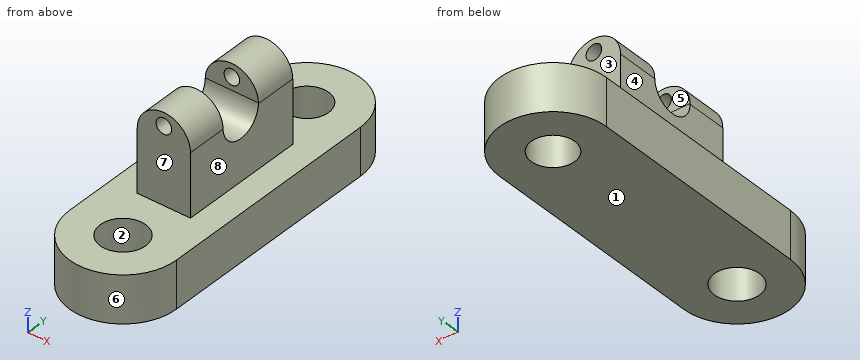
from build123d import *

# Parameters (mm, degrees)
F0_R      = 9.207917
F0_R_2    = 8.8097795002
F1_DEPTH  = 19.05
F2_W      = 21.5854309499
F2_H      = 51.5172295272
F3_DEPTH  = 25.4
F5_DEPTH  = 53.34
F7_DEPTH  = 25.4
F8_DEPTH  = 25.4
F9_W      = 17.8439589217
F9_H      = 25.0391028821
F10_DEPTH = 25.4
F11_DEPTH = 25.4
F12_R     = 3.1560406616
F13_DEPTH = 76.2


with BuildPart() as f1:
    # F0 (on Top) → F1 (new body)
    with BuildSketch(Plane.XY):
        with BuildLine():
            ThreePointArc((21.6257235091, 46.3394257879), (0, 67.965149297), (-21.6257235091, 46.3394257879))
            Line((-21.6257235091, 46.3394257879), (-21.6257235091, -46.3394257879))
            ThreePointArc((-21.6257235091, -46.3394257879), (0, -67.965149297), (21.6257235091, -46.3394257879))
            Line((21.6257235091, -46.3394257879), (21.6257235091, 46.3394257879))
        make_face()
        with Locations((0, -46.3394257879)):
            Circle(F0_R, mode=Mode.SUBTRACT)
        with Locations((0, 46.3394257879)):
            Circle(F0_R_2, mode=Mode.SUBTRACT)
    extrude(amount=F1_DEPTH)

    # F2 (on face) → F3 (join)
    with BuildSketch(Plane.XY.offset(19.05)):
        Rectangle(F2_W, F2_H)
    extrude(amount=F3_DEPTH)

    # F4 (on face) → F5 (join)
    with BuildSketch(Plane.XZ.offset(25.7586147636)):
        with BuildLine():
            Line((0, 44.45), (10.792715475, 44.45))
            ThreePointArc((10.792715475, 44.45), (0, 55.242715475), (-10.792715475, 44.45))
            Line((-10.792715475, 44.45), (0, 44.45))
        make_face()
    extrude(amount=-F5_DEPTH)

    # F6 (on Right) → F7 (cut)
    with BuildSketch(Plane.YZ):
        Polygon((25.7586147636, 59.1440834105), (25.7586147636, 44.753793627), (25.7586147636, 35.5440117419), (39.5732931793, 35.5440117419), (39.5732931793, 59.1440834105), align=None)
    extrude(amount=-F7_DEPTH, mode=Mode.SUBTRACT)

    # F6 (on Right) → F8 (cut)
    with BuildSketch(Plane.YZ):
        Polygon((25.7586147636, 59.1440834105), (25.7586147636, 44.753793627), (25.7586147636, 35.5440117419), (39.5732931793, 35.5440117419), (39.5732931793, 59.1440834105), align=None)
    extrude(amount=F8_DEPTH, mode=Mode.SUBTRACT)

    # F9 (on Right) → F10 (cut)
    with BuildSketch(Plane.YZ):
        with Locations((-0.4317085259, 57.2733450681)):
            Rectangle(F9_W, F9_H)
        with BuildLine():
            Line((8.490270935, 44.753793627), (-9.3536879867, 44.753793627))
            ThreePointArc((-9.3536879867, 44.753793627), (-0.4317085259, 35.8318141662), (8.490270935, 44.753793627))
        make_face()
    extrude(amount=-F10_DEPTH, mode=Mode.SUBTRACT)

    # F9 (on Right) → F11 (cut)
    with BuildSketch(Plane.YZ):
        with Locations((-0.4317085259, 57.2733450681)):
            Rectangle(F9_W, F9_H)
        with BuildLine():
            Line((8.490270935, 44.753793627), (-9.3536879867, 44.753793627))
            ThreePointArc((-9.3536879867, 44.753793627), (-0.4317085259, 35.8318141662), (8.490270935, 44.753793627))
        make_face()
    extrude(amount=F11_DEPTH, mode=Mode.SUBTRACT)

    # F12 (on face) → F13 (cut)
    with BuildSketch(Plane.XZ.offset(25.7586147636)):
        with Locations((0, 49.9343015254)):
            Circle(F12_R)
    extrude(amount=-F13_DEPTH, mode=Mode.SUBTRACT)


solid = f1.part
Model file for the job. Use its own axes, mm. Face numbers are marked on the shaded views. A direction names the side the tool comes from. Give positions to 0.01 mm unless a question says otherwise; leave off trailing zeros. Order: outer loops, then holes, each group sorted by start corner. A loop starts at its lowest first (then second) coordinate and runs counter-clockwise, first axis right, second up. Notation, with made-up numbers: (77, 56) - (126, 56) arc R19 cw to (126, 87) - close; hole circle Ø5 at (29.25, 21.5). An arc over 180 degrees is marked (long way). Write item = value, one per line. Start each with the question number.
1. Cut at D-D, the plane x = -6.5. List the corners of the cut face in (y, z).
2. Cut at B-B, the plane y = -53. List the corners of the cut face in (x, z).
3. Drop flat-ended pins along their axis: P1, Ø8, axis at x = 0, z = 49.93, coming from the -Y side; P2, Ø3, axis at x = 16, y = -43.5, coming from the -Z side; P3, Ø5, axis at x = -4, z = 50.5, coming from the +Y side; P4, Ø12.5, axis at y = 7.5, z = 34, coming from the -X side. Give the stop position or say it passes through.
4. Cut at A-A, the plane x = 0. List the corners of the cut face in (y, z).
5. Probe line 1 along Z through (x, y) = (0, 14); line 2 along Y through (x, z) = (0, 6.5); line 3 along Y through (x, z) = (0.5, 46.5). List the from-to ranges inside material, lowest first.
6. Which spindle directions (+Z, -Z, +X, -X, +Y, -Y) get a long thin tool onto all of the face, cutting with end or side? Do the marked faces 4, 5, 6, 7 and 8. Say none if no direction does.
7. Cut at C-C, the plane z = 7.5. List the corners of the cut face in (x, y).
8. Two-plate mould, pull along Y, no slides. Class the marked faces 1, 2 and 3: pulls with the +Y half, pulls with the -Y half, needs draft (parallel to the pull), parting line crosses it, or undercut.
Taken from the geometry:
q1.outline = (-66.97, 0) - (-52.86, 0) - (-52.86, 19.05) - (-66.97, 19.05) - close; (-39.82, 0) - (40.39, 0) - (40.39, 19.05) - (25.76, 19.05) - (25.76, 53.07) - (8.49, 53.07) - (8.49, 44.75) arc R8.92 cw to (-9.35, 44.75) - (-9.35, 53.07) - (-25.76, 53.07) - (-25.76, 19.05) - (-39.82, 19.05) - close; (52.29, 0) - (66.97, 0) - (66.97, 19.05) - (52.29, 19.05) - close
q2.outline = (-20.57, 0) - (-6.36, 0) - (-6.36, 19.05) - (-20.57, 19.05) - close; (6.36, 0) - (20.57, 0) - (20.57, 19.05) - (6.36, 19.05) - close
q3.P1 = -25.76
q3.P2 = 0
q3.P3 = 25.76
q3.P4 = -10.79
q4.outline = (-67.97, 0) - (-55.55, 0) - (-55.55, 19.05) - (-67.97, 19.05) - close; (-37.13, 0) - (37.53, 0) - (37.53, 19.05) - (25.76, 19.05) - (25.76, 46.78) - (8.49, 46.78) - (8.49, 44.75) arc R8.92 cw to (-9.35, 44.75) - (-9.35, 46.78) - (-25.76, 46.78) - (-25.76, 19.05) - (-37.13, 19.05) - close; (-25.76, 53.09) - (-9.35, 53.09) - (-9.35, 55.24) - (-25.76, 55.24) - close; (8.49, 53.09) - (25.76, 53.09) - (25.76, 55.24) - (8.49, 55.24) - close; (55.15, 0) - (67.97, 0) - (67.97, 19.05) - (55.15, 19.05) - close
q5.line_1 = 0 to 46.78, 53.09 to 55.24
q5.line_2 = -67.97 to -55.55, -37.13 to 37.53, 55.15 to 67.97
q5.line_3 = -25.76 to -9.35, 8.49 to 25.76
q6.face_4 = +Z, -X, +Y, -Y
q6.face_5 = +Z, +X, -X
q6.face_6 = +Z, -Z, -Y
q6.face_7 = +Z, +X, -X, -Y
q6.face_8 = +Z, +X, +Y, -Y
q7.outline = (-21.63, -46.34) arc R21.63 ccw to (21.63, -46.34) - (21.63, 46.34) arc R21.63 ccw to (-21.63, 46.34) - close; hole circle Ø18.42 at (0, -46.34); hole circle Ø17.62 at (0, 46.34)
q8.face_1 = needs draft
q8.face_2 = undercut
q8.face_3 = pulls with the +Y half
